Source: CAD feature listing. Evaluate the final solid. Frame: model axes, mm. A direction names the side the tool comes from. Give positions to 0.01 mm unless a question says otherwise; leave off trailing zeros. Loops run counter-clockwise (first coordinate to the right, second up) from the corner with the lowest first, then second, coordinate; pieces in that order, holes last. Notation, with made-up numbers: M 35.5,-40 L 92.5,-40 A20 ccw 92.5,-19 Z; hole C 3,39.25 d8. An arc over 180 degrees is marked long. Answer in a Markdown table with one row per item.
```python
from build123d import *

# Parameters (mm, degrees)
SKETCH_1_W          = 6.5
SKETCH_1_H          = 3
SKETCH_1_W_2        = 22.5
EXTRUDE_1_DEPTH     = 7
FILLET_3_R          = 3.5
CUT_EXTRUDE_1_REACH = 70.886
SKETCH_2_R          = 1.25
FILLET_4_R          = 1
FILLET_5_R          = 1


with BuildPart() as part:
    # Эскиз1 → Бобышка-Вытянуть1 (new body)
    with BuildSketch(Plane(origin=(0, 0, 0), x_dir=(1, 0, 0), z_dir=(0, 1, 0))):
        with Locations((3.25, 1.5)):
            Rectangle(SKETCH_1_W, SKETCH_1_H)
        Polygon((9.5, 21.5), (9.5, 24.5), (6.5, 24.5), (6.5, 3), (6.5, 0), (9.5, 0), align=None)
        with Locations((20.75, 23)):
            Rectangle(SKETCH_1_W_2, SKETCH_1_H)
        with Locations((43.25, 23)):
            Rectangle(SKETCH_1_W_2, SKETCH_1_H)
        Polygon((57.5, 24.5), (54.5, 24.5), (54.5, 21.5), (54.5, 0), (57.5, 0), (57.5, 3), align=None)
        with Locations((60.75, 1.5)):
            Rectangle(SKETCH_1_W, SKETCH_1_H)
    extrude(amount=EXTRUDE_1_DEPTH)

    # Скругление3
    fillet_3_edges = [part.edges().sort_by_distance(p)[0] for p in [
        (64, 0, -1.5),
        (64, 7, -1.5),
        (0, 0, -1.5),
        (0, 7, -1.5),
        (57.5, 3.5, -24.5),
        (6.5, 3.5, -24.5),
        (54.5, 3.5, -21.5),
        (9.5, 3.5, -21.5),
    ]]
    fillet(fillet_3_edges, radius=FILLET_3_R - 0.0001)  # a hair under: the kernel refuses the full size

    # Эскиз2 → Вырез-Вытянуть1 (cut, up to next)
    with BuildSketch(Plane.XY, mode=Mode.PRIVATE) as cut_extrude_1_sk1:
        with Locations((3.5, 3.5)):
            Circle(SKETCH_2_R)
    cut_extrude_1_tool1 = extrude(cut_extrude_1_sk1.sketch, amount=-CUT_EXTRUDE_1_REACH, mode=Mode.PRIVATE) & part.part
    # Эскиз2 → Вырез-Вытянуть1 (cut, up to next)
    with BuildSketch(Plane.XY, mode=Mode.PRIVATE) as cut_extrude_1_sk2:
        with Locations((60.5, 3.5)):
            Circle(SKETCH_2_R)
    cut_extrude_1_tool2 = extrude(cut_extrude_1_sk2.sketch, amount=-CUT_EXTRUDE_1_REACH, mode=Mode.PRIVATE) & part.part
    add(cut_extrude_1_tool1.solids().sort_by_distance((3.5, 3.5, 0))[0], mode=Mode.SUBTRACT)
    add(cut_extrude_1_tool2.solids().sort_by_distance((60.5, 3.5, 0))[0], mode=Mode.SUBTRACT)

    # Скругление4
    fillet_4_edges = [part.edges().sort_by_distance(p)[0] for p in [
        (6.5, 0, -12.00005),
        (57.5, 0, -12.00005),
        (57.5, 7, -12.00005),
        (59.00005, 7, -3),
        (32, 7, -24.5),
        (4.99995, 7, -3),
        (7.525096977, 7, -23.474903023),
        (56.474903023, 7, -23.474903023),
        (59.00005, 0, -3),
        (62.974903023, 1.025096977, -3),
        (62.974903023, 5.974903023, -3),
        (6.5, 7, -12.00005),
        (4.99995, 0, -3),
        (32, 0, -24.5),
        (7.525096977, 0, -23.474903023),
        (56.474903023, 0, -23.474903023),
        (1.025096977, 5.974903023, -3),
        (1.025096977, 1.025096977, -3),
    ]]
    fillet(fillet_4_edges, radius=FILLET_4_R)

    # Скругление5
    fillet_5_edges = [part.edges().sort_by_distance(p)[0] for p in [
        (54.5, 3.5, 0),
        (9.5, 3.5, 0),
    ]]
    fillet(fillet_5_edges, radius=FILLET_5_R)


solid = part.part
```
1) Section B-B, the plane x = 29. Return loops of the section in (y, z), then the cut area to 3 significant figures.
Reply:
| item | result |
|---|---|
| outline | M 0,-23.5 A1 ccw 1,-24.5 L 6,-24.5 A1 ccw 7,-23.5 L 7,-21.5 L 0,-21.5 Z |
| area | 20.6 mm² |
2) Pin query (flat end, axial travel): pin 1 Ø2 at (y, z) = (2, -16) entering from -X; pin 2 Ø4 at (x, y) = (60.5, 3.5) entering from -Z; pin 3 Ø1.5 at (y, z) = (4, -15.5) entering from +X. Return the tip coordinate at first contact, or that it passes through.
Reply:
| item | result |
|---|---|
| pin 1 | stops at x = 6.5 |
| pin 2 | stops at z = -3 |
| pin 3 | stops at x = 57.5 |
3) Pull-direction query (X, two-part tool) for faces 6 (the cylindrical face through (1, 5.95, -1.01)), 7 (the flat face through (9.5, 3, -9)), 8 (the cylindrical face through (61.69, 3.88, -1.48)), 9 (the flat face through (32, 3, -24.5)); classes: released by +X, released by -X, zero draft, split by the parting line, or undercut.
Reply:
| item | result |
|---|---|
| face 6 | released by -X |
| face 7 | undercut |
| face 8 | undercut |
| face 9 | zero draft |
4) Set-up query: faces 1 (the cylindrical face through (4.077, 2.391, -1.479)), 2 (the flat face through (54.5, 3, -10)), 3 (the flat face through (6.5, 3, -12)), 4 (the cylindrical face through (1, 1.05, -1.01)), 5 (the flat face through (57.5, 3, -12)). Return all of +Z, -Z, +X, -X, +Y, -Y with unobstructed straight access to the full face (end or side cutting, diameter ignored); none if empty.
Reply:
| item | result |
|---|---|
| face 1 | +Z, -Z |
| face 2 | +Z, +Y, -Y |
| face 3 | -Z, -X, +Y, -Y |
| face 4 | +Z, -Z, -X, -Y |
| face 5 | -Z, +X, +Y, -Y |
5) Material intervals for L1, parallel to X at y = 3.75, z = -5.5; L2, parallel to Y at x = 3.5, z = -1.95; L3, parallel to Z at x = 37, y = 2.5, sorted ascending.
Reply:
| item | result |
|---|---|
| L1 | x = 6.5 to 9.5, 54.5 to 57.5 |
| L2 | y = 0 to 2.25, 4.75 to 7 |
| L3 | z = -24.5 to -21.5 |
6) Section A-A, the plane z = -12.25. Return loops of the section in (x, y), then the cut area to 3 significant figures.
Reply:
| item | result |
|---|---|
| outline | M 6.5,1 A1 ccw 7.5,0 L 9.5,0 L 9.5,7 L 7.5,7 A1 ccw 6.5,6 Z; M 54.5,0 L 56.5,0 A1 ccw 57.5,1 L 57.5,6 A1 ccw 56.5,7 L 54.5,7 Z |
| area | 41.1 mm² |
